```python
from build123d import *

# Parameters (mm, degrees)
BOSS_EXTRUDE1_DEPTH = 20
FILLET1_R           = 6
SKETCH5_W           = 7
SKETCH5_H           = 15
BOSS_EXTRUDE3_DEPTH = 2
CUT_EXTRUDE1_DEPTH  = 5
SKETCH3_R           = 9.5
CUT_EXTRUDE2_DEPTH  = 7
SKETCH6_W           = 7
SKETCH6_H           = 15
BOSS_EXTRUDE4_DEPTH = 2
FILLET3_R           = 4
FILLET2_R           = 10
CHAMFER1_SIZE       = 2


# Some blends are built 0.0001 mm under size
with BuildPart() as part:
    # Sketch1 → Boss-Extrude1 (new body)
    with BuildSketch(Plane.XY):
        Polygon((-37.553334028, 5.009990716), (-37.553334028, 0.009990716), (-137.553334028, 0.009990716), (-142.053334028, -4.490009284), (-142.053334028, -54.490009284), (-149.053334028, -54.490009284), (-149.053334028, -1.590514347), (-142.452828965, 5.009990716), align=None)
    extrude(amount=BOSS_EXTRUDE1_DEPTH)

    # Fillet1
    fillet1_edges = [part.edges().sort_by_distance(p)[0] for p in [
        (-137.553334028, 0.009990716, 10),
        (-142.053334028, -4.490009284, 10),
    ]]
    fillet(fillet1_edges, radius=FILLET1_R)

    # Sketch5 → Boss-Extrude3 (add)
    with BuildSketch(Plane.XY.offset(20)):
        with Locations((-145.553334028, -37.485290658)):
            Rectangle(SKETCH5_W, SKETCH5_H)
    extrude(amount=BOSS_EXTRUDE3_DEPTH)

    # Sketch2 → Cut-Extrude1 (cut)
    with BuildSketch(Plane(origin=(0, 0.009990716, 0), x_dir=(-1, 0, 0), z_dir=(0, -1, 0))):
        with BuildLine():
            Line((125.068052654, -11.1), (47.553334028, -11.1))
            ThreePointArc((47.553334028, -11.1), (46.453334028, -10), (47.553334028, -8.9))
            Line((47.553334028, -8.9), (125.068052654, -8.9))
            ThreePointArc((125.068052654, -8.9), (126.168052654, -10), (125.068052654, -11.1))
        make_face()
        with BuildLine():
            Line((125.068052654, -3.9), (47.553334028, -3.9))
            ThreePointArc((47.553334028, -3.9), (46.453334028, -5), (47.553334028, -6.1))
            Line((47.553334028, -6.1), (125.068052654, -6.1))
            ThreePointArc((125.068052654, -6.1), (126.168052654, -5), (125.068052654, -3.9))
        make_face()
        with BuildLine():
            Line((125.068052654, -16.1), (47.553334028, -16.1))
            ThreePointArc((47.553334028, -16.1), (46.453334028, -15), (47.553334028, -13.9))
            Line((47.553334028, -13.9), (125.068052654, -13.9))
            ThreePointArc((125.068052654, -13.9), (126.168052654, -15), (125.068052654, -16.1))
        make_face()
    extrude(amount=-CUT_EXTRUDE1_DEPTH, mode=Mode.SUBTRACT)

    # Sketch3 → Cut-Extrude2 (cut)
    with BuildSketch(Plane(origin=(-142.053334028, 0, 0), x_dir=(0, 0, -1), z_dir=(1, 0, 0))):
        with Locations((-10, -37.485290658)):
            Circle(SKETCH3_R)
    extrude(amount=-CUT_EXTRUDE2_DEPTH, mode=Mode.SUBTRACT)

    # Sketch6 → Boss-Extrude4 (add)
    with BuildSketch(Plane(origin=(0, 0, 0), x_dir=(-1, 0, 0), z_dir=(0, 0, -1))):
        with Locations((145.553334028, -37.485290658)):
            Rectangle(SKETCH6_W, SKETCH6_H)
    extrude(amount=BOSS_EXTRUDE4_DEPTH)

    # Fillet3
    # the kernel refuses this fillet: 4 mm, written as the material it takes off along each edge
    with BuildSketch(Plane(origin=(-37.553334028, 5.009990716, -10), x_dir=(0, -1, 0), z_dir=(0, 0, 1)), Plane(origin=(-37.553334028, 0.009990716, -10), x_dir=(-1, 0, 0), z_dir=(0, 0, 1))) as fillet3_piece_1:
        with BuildLine():
            CenterArc((FILLET3_R, -FILLET3_R), FILLET3_R, 90, 90)
            Line((0, -FILLET3_R), (0, 0))
            Line((0, 0), (FILLET3_R, 0))
        make_face()
    extrude(amount=40, mode=Mode.SUBTRACT)

    # Fillet2
    fillet2_edges = [part.edges().sort_by_distance(p)[0] for p in [
        (-149.053334028, -1.590514347, 10),
        (-142.452828965, 5.009990716, 10),
    ]]
    fillet(fillet2_edges, radius=FILLET2_R)

    # Chamfer1
    chamfer1_edges = [part.edges().sort_by_distance(p)[0] for p in [
        (-145.553334028, -29.985290658, 22),
        (-145.553334028, -44.985290658, 22),
        (-145.553334028, -29.985290658, -2),
        (-145.553334028, -44.985290658, -2),
    ]]
    chamfer(chamfer1_edges, length=CHAMFER1_SIZE - 0.0001)  # a hair under: the kernel refuses the full size


solid = part.part
```
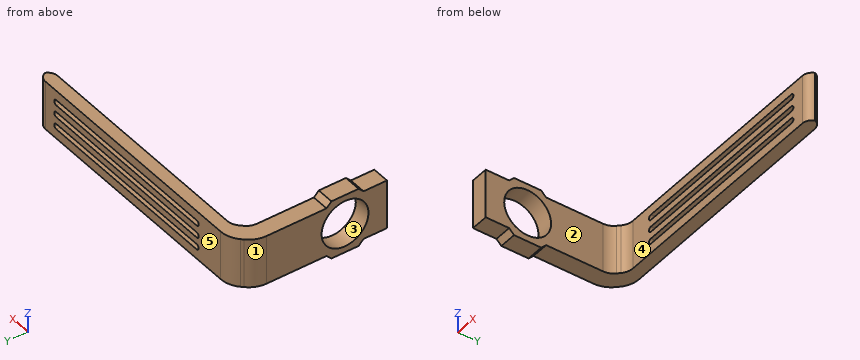
For this review, take the finished solid that the model builds, in its own axes (mm). Face numbers are marked on the shaded views. A direction names the side the tool comes from. Round coordinates to 2 decimals unless told otherwise and drop trailing zeros. Write each loop counter-clockwise with the first axis right and the second up, starting at its lowest first coordinate (ties: lowest second). Pieces come first, ordered by that corner, then holes. Notation, with made-up numbers: (86, 25.25) - (122, 25.25) arc R29 cw to (122, 59.25) - close; hole circle Ø10 at (69.25, 52). An arc over 180 degrees is marked (long way). Put each result on its own line as item: value.
Q1. We need section A-A (z = 10). Give the boundary of the cut face in (x, y), and give its area (3 significant figures).
Solved:
outline: (-149.05, -54.49) - (-142.05, -54.49) - (-142.05, -46.99) - (-149.05, -46.99) - close; (-149.05, -27.99) - (-142.05, -27.99) - (-142.05, -6.98) arc R6 cw to (-140.3, -2.73) - (-139.31, -1.75) arc R6 cw to (-135.07, 0.01) - (-126.17, 0.01) - (-126.17, 5.01) - (-138.31, 5.01) arc R10 ccw to (-145.38, 2.08) - (-146.12, 1.34) arc R10 ccw to (-149.05, -5.73) - close; (-46.45, 0.01) - (-41.55, 0.01) arc R4 ccw to (-37.85, 2.51) arc R4 ccw to (-41.55, 5.01) - (-46.45, 5.01) - close
area: 386 mm2
Q2. Machinability: for the marked faces 4 and 5, which of the approach directions +Z, -Z, +X, -X, +Y, -Y give a long, thin tool a straight path to every point of the face, cutting with its end or side? Answer none if there is none.
Solved:
face 4: +Z, -Z, +X, -Y
face 5: +Z, -Z, +X, -X, +Y
Q3. We need section D-D (z = 5). Give the boundary of the cut face in (x, y).
Solved:
outline: (-149.05, -54.49) - (-142.05, -54.49) - (-142.05, -45.56) - (-149.05, -45.56) - close; (-149.05, -29.41) - (-142.05, -29.41) - (-142.05, -6.98) arc R6 cw to (-140.3, -2.73) - (-139.31, -1.75) arc R6 cw to (-135.07, 0.01) - (-126.17, 0.01) - (-126.17, 5.01) - (-138.31, 5.01) arc R10 ccw to (-145.38, 2.08) - (-146.12, 1.34) arc R10 ccw to (-149.05, -5.73) - close; (-46.45, 0.01) - (-41.55, 0.01) arc R4 ccw to (-37.85, 2.51) arc R4 ccw to (-41.55, 5.01) - (-46.45, 5.01) - close
Q4. We need section C-C (y = -41). Give the boundary of the cut face in (x, z), and give its area (3 significant figures).
Solved:
outline: (-149.05, -2) - (-142.05, -2) - (-142.05, 1.17) - (-149.05, 1.17) - close; (-149.05, 18.83) - (-142.05, 18.83) - (-142.05, 22) - (-149.05, 22) - close
area: 44.4 mm2
Q5. Mouldability with a two-part tool opening along Y and no side actions: class the marked faces 1, 2 and 3 as released by +Y, released by -Y, zero draft, split by the parting line, or undercut.
Solved:
face 1: released by +Y
face 2: zero draft
face 3: undercut
Q6. Wall thickness on probe 1 along Z at (x, y) = (-104, 2); probe 2 along X at (y, z) = (-30, 3.75); probe 3 along Y at (x, z) = (-59, 0.25): over which ranges is each line inside the solid? List them lowest first.
Solved:
probe 1: z = 0 to 3.9, 6.1 to 8.9, 11.1 to 13.9, 16.1 to 20
probe 2: x = -149.05 to -142.05
probe 3: y = 0.01 to 5.01
Q7. We need section B-B (x = -61). Give the boundary of the cut face in (y, z).
Solved:
outline: (0.01, 0) - (5.01, 0) - (5.01, 3.9) - (0.01, 3.9) - close; (0.01, 6.1) - (5.01, 6.1) - (5.01, 8.9) - (0.01, 8.9) - close; (0.01, 11.1) - (5.01, 11.1) - (5.01, 13.9) - (0.01, 13.9) - close; (0.01, 16.1) - (5.01, 16.1) - (5.01, 20) - (0.01, 20) - close
Q8. Insertion check: pin 1 Ø5.5 at (x, y) = (-84.5, 2.5) entering from +Z; pin 2 Ø5 at (x, z) = (-87.5, 14) entering from -Y; pin 3 Ø5.5 at (x, y) = (-81, 2.5) entering from -Z. Each pin has a flat end and moves straight along its axis. Give the tip position at first contact, or say it passes through.
Solved:
pin 1: stops at z = 20
pin 2: stops at y = 0.01
pin 3: stops at z = 0
